Geometry check sheet. Reference: the model listing, model coordinates, mm. A direction names the side the tool comes from. Round coordinates to 2 decimals unless told otherwise and drop trailing zeros. Loops run counter-clockwise (first coordinate to the right, second up) from the corner with the lowest first, then second, coordinate; pieces in that order, holes last.
```python
from build123d import *

# Parameters (mm, degrees)
F1_DEPTH = 55
F3_DEPTH = 44.001
F4_R     = 4
F5_DEPTH = 43.501


with BuildPart() as f1:
    # F0 (on Top) → F1 (new body)
    with BuildSketch(Plane.XY):
        with BuildLine():
            Line((51.874786, -31.5), (51.874786, 33.5))
            Line((51.874786, 33.5), (31.374786, 33.5))
            Line((31.374786, 33.5), (31.374786, 12.5))
            Line((31.374786, 12.5), (8.374786, 12.5))
            Line((8.374786, 12.5), (8.374786, 2))
            Line((8.374786, 2), (25.289246, 2))
            ThreePointArc((25.289246, 2), (32.653455, 1), (25.289246, 0))
            Line((25.289246, 0), (8.374786, 0))
            Line((8.374786, 0), (8.374786, -10.5))
            Line((8.374786, -10.5), (31.374786, -10.5))
            Line((31.374786, -10.5), (31.374786, -31.5))
            Line((31.374786, -31.5), (51.874786, -31.5))
        make_face()
    extrude(amount=F1_DEPTH)

    # F2 (on face) → F3 (cut, through all)
    with BuildSketch(Plane.XZ.offset(10.5)):
        with BuildLine():
            ThreePointArc((13.374786, 44.981502), (17.374786, 40.981502), (21.374786, 44.981502))
            ThreePointArc((21.374786, 44.981502), (17.374786, 48.981502), (13.374786, 44.981502))
        make_face()
        with BuildLine():
            ThreePointArc((13.374786, 10), (17.374786, 6), (21.374786, 10))
            ThreePointArc((21.374786, 10), (17.374786, 14), (13.374786, 10))
        make_face()
    extrude(amount=-F3_DEPTH, mode=Mode.SUBTRACT)

    # F4 (on face) → F5 (cut, through all)
    with BuildSketch(Plane.YZ.offset(51.874786)):
        with BuildLine():
            ThreePointArc((-26.5, 45), (-22.5, 41), (-18.5, 45))
            ThreePointArc((-18.5, 45), (-22.5, 49), (-26.5, 45))
        make_face()
        with Locations((24.5, 45)):
            Circle(F4_R)
        with Locations((24.5, 10)):
            Circle(F4_R)
        with BuildLine():
            ThreePointArc((-25.441907, 10), (-21.441907, 6), (-17.441907, 10))
            ThreePointArc((-17.441907, 10), (-21.441907, 14), (-25.441907, 10))
        make_face()
    extrude(amount=-F5_DEPTH, mode=Mode.SUBTRACT)


solid = f1.part
```
1) Sectioned sample at B-B, the plane x = 41. Record the cut outline in (y, z).
Report:
outline: (-31.5, 0) - (33.5, 0) - (33.5, 55) - (-31.5, 55) - close; hole circle Ø8 at (-22.5, 45); hole circle Ø8 at (-21.44, 10); hole circle Ø8 at (24.5, 10); hole circle Ø8 at (24.5, 45)
2) Gauge pin test, flat ends, axial feed: pin 1 (7 mm diameter, centred on x = 17.37, z = 44.98, fed in from +Y); pin 2 (12 mm diameter, centred on x = 29.5, y = -21, fed in from +Z); pin 3 (18.5 mm diameter, centred on x = 15.5, z = 22.5, fed in from -Y); pin 4 (8.5 mm diameter, centred on x = 17, z = 14.5, fed in from +Y). Record the tip position at first contact, or that the pin passes through.
Report:
pin 1: passes through
pin 2: stops at z = 55
pin 3: stops at y = -10.5
pin 4: stops at y = 12.5
3) Sectioned sample at C-C, the plane z = 11.5. Record the cut outline in (x, y).
Report:
outline: (8.37, -10.5) - (13.67, -10.5) - (13.67, 0) - (8.37, 0) - close; (8.37, 2) - (13.67, 2) - (13.67, 12.5) - (8.37, 12.5) - close; (21.08, -10.5) - (31.37, -10.5) - (31.37, -17.73) - (51.87, -17.73) - (51.87, 20.79) - (31.37, 20.79) - (31.37, 12.5) - (21.08, 12.5) - (21.08, 2) - (25.29, 2) arc R3.75 cw (long way) to (25.29, 0) - (21.08, 0) - close; (31.37, -31.5) - (51.87, -31.5) - (51.87, -25.15) - (31.37, -25.15) - close; (31.37, 28.21) - (51.87, 28.21) - (51.87, 33.5) - (31.37, 33.5) - close
4) Mould release check, pull along X, two halves, no side actions. Record for faces 1 (the face through (41.768, -17.627, 11.201)), 2 (the face through (32.65, 1.15, 27.12)), 3 (the face through (31.375, -21, 27)): +X half, -X half, draft (parallel to the pull), parting line (faces both ways), or undercut.
Report:
face 1: draft
face 2: undercut
face 3: -X half
5) Access from +Z, -Z, +X, -X, +Y, -Y to the whole of each face (thin tool, end or side, straight path). Record for faces 4 (the face through (17, 2, 27)), 5 (the face through (20, 12.5, 27)), 6 (the face through (8.375, -5, 27)), 7 (the face through (20, -10.5, 27)), 8 (the face through (42, 33.5, 27)).
Report:
face 4: +Z, -Z, -X
face 5: +Z, -Z, -X, +Y
face 6: +Z, -Z, -X, +Y, -Y
face 7: +Z, -Z, -X, -Y
face 8: +Z, -Z, +X, -X, +Y
6) Scan lines: line 1 along Y through (x, z) = (15.5, 23.5); line 2 along Z through (x, y) = (31.5, 28); line 3 along Y through (x, z) = (49, 44.5). Record each from-to range of solid material in increasing order.
Report:
line 1: y = -10.5 to 0, 2 to 12.5
line 2: z = 0 to 8.06, 11.94 to 43.06, 46.94 to 55
line 3: y = -31.5 to -26.47, -18.53 to 20.53, 28.47 to 33.5
7) Sectioned sample at D-D, the plane z = 23. Record the cut outline in (x, y).
Report:
outline: (8.37, -10.5) - (31.37, -10.5) - (31.37, -31.5) - (51.87, -31.5) - (51.87, 33.5) - (31.37, 33.5) - (31.37, 12.5) - (8.37, 12.5) - (8.37, 2) - (25.29, 2) arc R3.75 cw (long way) to (25.29, 0) - (8.37, 0) - close
8) Sectioned sample at A-A, the plane y = 24.5. Record the cut outline in (x, z), then the cut area to 4 significant figures.
Report:
outline: (31.37, 0) - (51.87, 0) - (51.87, 6) - (31.37, 6) - close; (31.37, 14) - (51.87, 14) - (51.87, 41) - (31.37, 41) - close; (31.37, 49) - (51.87, 49) - (51.87, 55) - (31.37, 55) - close
area: 799.5 mm2
